```python
from build123d import *

# Parameters (mm, degrees)
SKETCH1_R           = 140.65
BOSS_EXTRUDE1_DEPTH = 12.7
BOSS_EXTRUDE2_DEPTH = 72.4
CIRPATTERN1_COUNT   = 16
SKETCH4_R           = 140.65
CUT_EXTRUDE1_DEPTH  = 12.7


with BuildPart() as part:
    # Sketch1 → Boss-Extrude1 (new body)
    with BuildSketch(Plane(origin=(0, 0, 0), x_dir=(1, 0, 0), z_dir=(0, 1, 0))):
        with Locations(Location((0, 0, 0), (0, 0, 270))):
            Circle(SKETCH1_R)
    extrude(amount=BOSS_EXTRUDE1_DEPTH)

    # Sketch3 → Boss-Extrude2 (add)
    with BuildSketch(Plane(origin=(0, 12.7, 0), x_dir=(1, 0, 0), z_dir=(0, 1, 0))):
        Polygon((-62.512510333, 104.73288314), (-16.28303914, 123.781137474), (-23.902340873, 142.272925951), (-70.131812067, 123.224671617), align=None)
    boss_extrude2 = extrude(amount=BOSS_EXTRUDE2_DEPTH)

    # CirPattern1: Boss-Extrude2 ×16 about axis
    cirpattern1_axis = Axis((0.678796416, 0, 1.91510031), (0, 1, 0))
    for i in range(1, CIRPATTERN1_COUNT):
        add(boss_extrude2.rotate(cirpattern1_axis, i * 360 / CIRPATTERN1_COUNT))

    # Sketch4 → Cut-Extrude1 (cut)
    with BuildSketch(Plane.XZ):
        Circle(SKETCH4_R)
    extrude(amount=-CUT_EXTRUDE1_DEPTH, mode=Mode.SUBTRACT)


solid = part.part
```
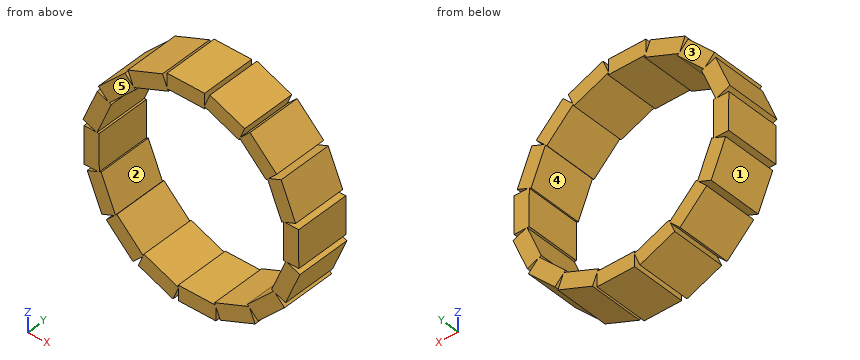
Input: part model. Units: mm. Frame: model coordinates. Face numbers are marked on the shaded views. A direction names the side the tool comes from. Coordinates: 2 decimals unless noted, no trailing zeros. Loops run counter-clockwise (first coordinate to the right, second up) from the corner with the lowest first, then second, coordinate; pieces in that order, holes last. Notation, with made-up numbers: M 23,6 L 38,6 A10 cw 38,17 Z; hole C 67.5,65 d4. An arc over 180 degrees is marked long. One line per item, written item: value.
(1) Pin query (flat end, axial travel): pin 1 (3 mm diameter, centred on x = 112, y = 59, fed in from +Z); pin 2 (5 mm diameter, centred on x = -105.5, y = 71, fed in from -Z); pin 3 (10 mm diameter, centred on x = 36.5, y = 67.5, fed in from -Z). Return the tip coordinate at first contact, or that it passes through.
Filled in:
pin 1: z = 93.91
pin 2: z = -96.2
pin 3: z = -140.71
(2) Section B-B (x = -5). Output: boundary loops of the cut face in (y, z), and give its area (3 significant figures).
Filled in:
outline: M 12.7,-140.77 L 85.1,-140.77 L 85.1,-120.77 L 12.7,-120.77 Z; M 12.7,124.58 L 85.1,124.58 L 85.1,144.58 L 12.7,144.58 Z
area: 2,900 mm^2
(3) Line query: line 1 along X through (y, z) = (30, -5.5); line 2 along X through (y, z) = (50, 125.5); line 3 along Z through (x, y) = (78.5, 77). Output: solid intervals per line, ascending. Write a range as from..to.
Filled in:
line 1: -141.99..-121.99, 123.37..143.37
line 2: -73.7..18.25, 22.76..70.85, 78.35..78.79
line 3: -120.23..-101.2, -100.74..-93.79, 97.56..125.65
(4) Pull-direction query (X, two-part tool) for the marked faces 1, 2 and 3; classes: +X half, -X half, draft (parallel to the pull), parting line (faces both ways), or undercut.
Filled in:
face 1: -X half
face 2: undercut
face 3: draft
(5) Reachability of the marked faces 4 and 5 from +Z, -Z, +X, -X, +Y, -Y: full face, straight path, thin tool, end or side. Return the list, or none.
Filled in:
face 4: +Y, -Y
face 5: +Z, -Z, +X, -X, -Y
(6) Section A-A (z = -93). Output: boundary loops of the cut face in (x, y), and give its area (3 significant figures).
Filled in:
outline: M -106.21,12.7 L -77.87,12.7 L -77.87,85.1 L -106.21,85.1 Z; M 79.29,12.7 L 107.52,12.7 L 107.52,85.1 L 79.29,85.1 Z
area: 4,100 mm^2
